Print and shaded views of the part. All mm, measured from the part's lowest x, y and z. A direction names the side the tool comes from. Give positions to 0.01 mm unless a question says otherwise; leave off trailing zeros. Loops run counter-clockwise (first coordinate to the right, second up) from the corner with the lowest first, then second, coordinate; pieces in that order, holes last.
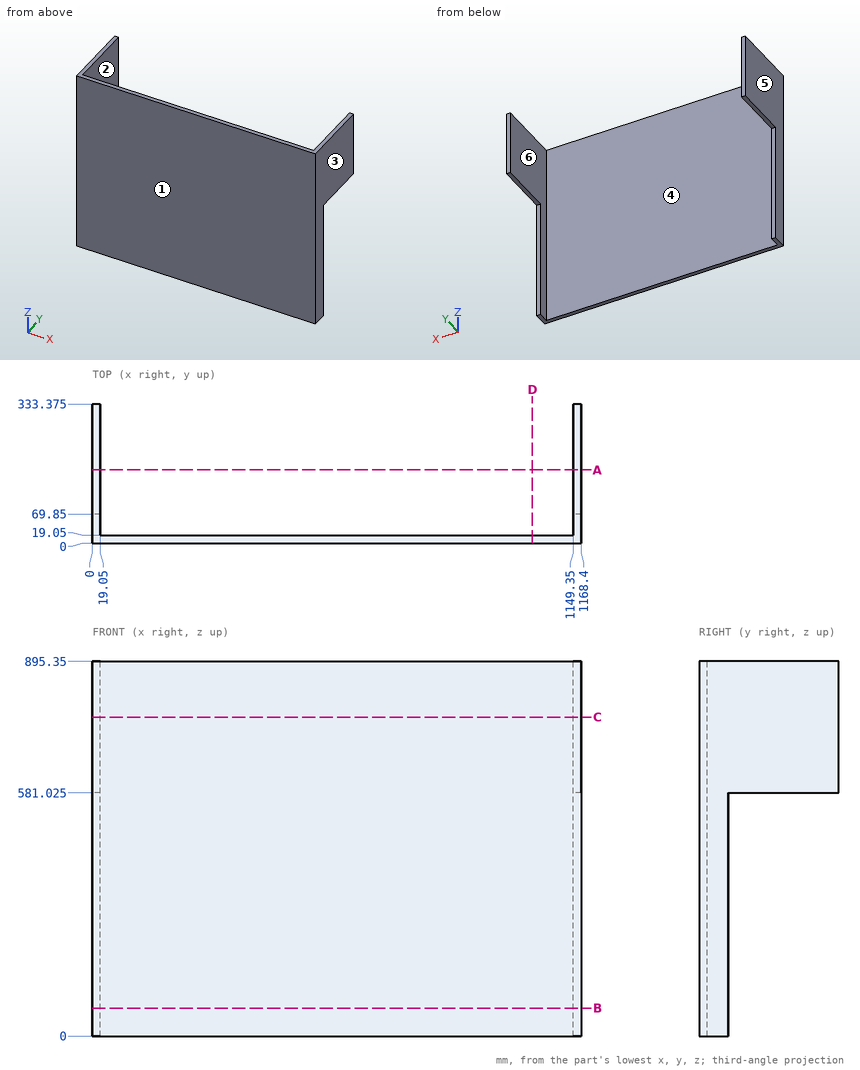
1. Drop flat-ended pins along their axis: pin 1 (8 mm diameter, centred on x = 631, z = 516, fed in from +Y); pin 2 (21 mm diameter, centred on x = 1156.5, y = 241, fed in from -Z) (3 decimals); pin 3 (9.5 mm diameter, centred on x = 14, z = 354, fed in from +Y). Give the stop position or say it passes through.
Responses:
pin 1: stops at y = 19.05
pin 2: stops at z = 581.025
pin 3: stops at y = 69.85
2. Saw through at C-C, the plane z = 762. List the corners of the cut face in (x, y) (3 decimals), and give its area (3 significant figures).
Responses:
outline: (0, 0) - (1168.4, 0) - (1168.4, 333.375) - (1149.35, 333.375) - (1149.35, 19.05) - (19.05, 19.05) - (19.05, 333.375) - (0, 333.375) - close
area: 34,200 mm2
3. Saw through at B-B, the plane z = 66.5. List the corners of the cut face in (x, y), and give its area (3 significant figures).
Responses:
outline: (0, 0) - (1168.4, 0) - (1168.4, 69.85) - (1149.35, 69.85) - (1149.35, 19.05) - (19.05, 19.05) - (19.05, 69.85) - (0, 69.85) - close
area: 24,200 mm2
4. Pull direction X, two halves, no side cores. Call the marked faces 1, 2, 3 and 4: released by +X, released by -X, zero draft, split by the parting line, or undercut.
Responses:
face 1: zero draft
face 2: undercut
face 3: released by +X
face 4: undercut
5. Saw through at A-A, the plane y = 176. List the corners of the cut face in (x, z) (3 decimals).
Responses:
outline: (0, 581.025) - (19.05, 581.025) - (19.05, 895.35) - (0, 895.35) - close; (1149.35, 581.025) - (1168.4, 581.025) - (1168.4, 895.35) - (1149.35, 895.35) - close
6. Probe line 1 along X through (y, z) = (99, 647.5); line 2 along Y through (x, z) = (430, 373). List the from-to ranges inside material, lowest first.
Responses:
line 1: x = 0 to 19.05, 1149.35 to 1168.4
line 2: y = 0 to 19.05
7. Tool access for the marked faces 5 and 6: list every direction of +Z, -Z, +X, -X, +Y, -Y with a clear straight run to the whole face (end or side of a thin tool).
Responses:
face 5: +Z, -Z, -X, +Y, -Y
face 6: +Z, -Z, +Y
8. Saw through at D-D, the plane x = 1052. List the corners of the cut face in (y, z), and give its area (3 significant figures).
Responses:
outline: (0, 0) - (19.05, 0) - (19.05, 895.35) - (0, 895.35) - close
area: 17,100 mm2
